from build123d import *

# Parameters (mm, degrees)
F0_W      = 368.3
F0_H      = 50.8
F1_DEPTH  = 38.1
F2_W      = 76.2
F2_H      = 50.8
F3_DEPTH  = 38.1
F4_W      = 3.175
F4_H      = 63.5
F5_DEPTH  = 12.7
F6_W      = 44.45
F6_H      = 50.8
F7_DEPTH  = 38.1
F8_R      = 2.54
F9_DEPTH  = 12.7
F10_W     = 76.2
F10_H     = 6.35
F10_W_2   = 38.1
F11_DEPTH = 76.2


with BuildPart() as f1:
    # F0 (on Right) → F1 (new body)
    with BuildSketch(Plane.YZ):
        with Locations((184.15, 25.4)):
            Rectangle(F0_W, F0_H)
    extrude(amount=F1_DEPTH)

    # F2 (on face) → F3 (join)
    with BuildSketch(Plane.YZ.offset(38.1)):
        with Locations((38.1, 25.4)):
            Rectangle(F2_W, F2_H)
        with Locations((330.2, 25.4)):
            Rectangle(F2_W, F2_H)
    extrude(amount=F3_DEPTH)

    # F4 (on face) → F5 (cut)
    with BuildSketch(Plane.XY.offset(50.8)):
        with Locations((13.5509, 38.1)):
            Rectangle(F4_W, F4_H)
        with Locations((13.5509, 330.2)):
            Rectangle(F4_W, F4_H)
        Polygon((10.905067, 69.85), (11.9634, 69.85), (15.1384, 69.85), (15.1384, 298.45), (11.9634, 298.45), (10.905067, 298.45), align=None)
    extrude(amount=-F5_DEPTH, mode=Mode.SUBTRACT)

    # F6 (on face) → F7 (cut)
    with BuildSketch(Plane.XY.offset(50.8)):
        with Locations((47.625, 38.1)):
            Rectangle(F6_W, F6_H)
        with Locations((47.625, 330.2)):
            Rectangle(F6_W, F6_H)
    extrude(amount=-F7_DEPTH, mode=Mode.SUBTRACT)

    # F8 (on face) → F9 (cut)
    with BuildSketch(Plane.YZ.offset(38.1)):
        with Locations((120.65, 25.4)):
            Circle(F8_R)
        with Locations((146.05, 25.4)):
            Circle(F8_R)
        with Locations((171.45, 25.4)):
            Circle(F8_R)
        with Locations((196.85, 25.4)):
            Circle(F8_R)
        with Locations((222.25, 25.4)):
            Circle(F8_R)
        with Locations((247.65, 25.4)):
            Circle(F8_R)
        with Locations((95.25, 25.4)):
            Circle(F8_R)
        with Locations((273.05, 25.4)):
            Circle(F8_R)
    extrude(amount=-F9_DEPTH, mode=Mode.SUBTRACT)

    # F10 (on face) → F11 (cut)
    with BuildSketch(Plane.XY.offset(50.8)):
        with Locations((38.1, 3.175)):
            Rectangle(F10_W, F10_H)
        with Locations((57.15, 73.025)):
            Rectangle(F10_W_2, F10_H)
        with Locations((38.1, 365.125)):
            Rectangle(F10_W, F10_H)
        with Locations((57.15, 295.275)):
            Rectangle(F10_W_2, F10_H)
    extrude(amount=-F11_DEPTH, mode=Mode.SUBTRACT)


solid = f1.part
CAD build for the part. Positions are in the model's coordinates, mm. A direction names the side the tool comes from. Coordinates: 2 decimals unless noted, no trailing zeros. Order: outer loops, then holes, each group sorted by start corner. A loop starts at its lowest first (then second) coordinate and runs counter-clockwise, first axis right, second up. Notation, with made-up numbers: (-7.5, 43.25) -> (-2.5, 43.25) arc R7 cw to (-2.5, 55.25) -> close; hole circle Ø11 at (56, 49.25). An arc over 180 degrees is marked (long way). Answer in a Markdown table with one row per item.
1) Band-saw the part on B-B (y = 29). List the corners of the cut face in (x, z).
Check values:
| item | result |
|---|---|
| outline | (0, 0) -> (76.2, 0) -> (76.2, 50.8) -> (69.85, 50.8) -> (69.85, 12.7) -> (25.4, 12.7) -> (25.4, 50.8) -> (15.14, 50.8) -> (15.14, 38.1) -> (11.96, 38.1) -> (11.96, 50.8) -> (0, 50.8) -> close |
2) Mould opens along Y. For faces 1 (the face through (11.963, 330, 45)), 2 (the face through (38, 361.95, 26)), 3 (the face through (10.905, 186, 45)) say: pulls with the +Y half, pulls with the -Y half, needs draft (parallel to the pull), parting line crosses it, or undercut.
Check values:
| item | result |
|---|---|
| face 1 | needs draft |
| face 2 | pulls with the +Y half |
| face 3 | undercut |
3) Drill centre lines: line 1 (Y direction, x = 40, z = 24.5); line 2 (Y direction, x = 25.5, z = 46.5); line 3 (Z direction, x = 35.75, y = 120.65). Where is each one in solid material? Low to high.
Check values:
| item | result |
|---|---|
| line 1 | 6.35 to 12.7, 63.5 to 69.85, 298.45 to 304.8, 355.6 to 361.95 |
| line 2 | 6.35 to 12.7, 63.5 to 304.8, 355.6 to 361.95 |
| line 3 | 0 to 22.86, 27.94 to 50.8 |
4) Which spindle directions (+Z, -Z, +X, -X, +Y, -Y) get a long thin tool onto all of the face, cutting with end or side? Do faces 4 (the face through (47, 355.6, 32)), 5 (the face through (6, 182, 50.8)), 6 (the face through (38.1, 183, 26)). Say none if no direction does.
Check values:
| item | result |
|---|---|
| face 4 | +Z |
| face 5 | +Z, +X, -X, +Y, -Y |
| face 6 | +Z, -Z, +X |
5) Band-saw the part on A-A (x = 48.5). List the corners of the cut face in (y, z), and give its area (3 significant figures).
Check values:
| item | result |
|---|---|
| outline | (6.35, 0) -> (69.85, 0) -> (69.85, 50.8) -> (63.5, 50.8) -> (63.5, 12.7) -> (12.7, 12.7) -> (12.7, 50.8) -> (6.35, 50.8) -> close; (298.45, 0) -> (361.95, 0) -> (361.95, 50.8) -> (355.6, 50.8) -> (355.6, 12.7) -> (304.8, 12.7) -> (304.8, 50.8) -> (298.45, 50.8) -> close |
| area | 2,580 mm2 |
6) Flat gauge pins, fed straight in: P1, Ø5.5, axis at y = 121.5, z = 26, coming from the +X side; P2, Ø1.5, axis at x = 35, y = 48, coming from the +Z side; P3, Ø3, axis at y = 171.45, z = 25.4, coming from the +X side. Where does each tip first touch, or does it go through?
Check values:
| item | result |
|---|---|
| P1 | x = 38.1 |
| P2 | z = 12.7 |
| P3 | x = 25.4 |
7) Band-saw the part on C-C (y = 295). List the corners of the cut face in (x, z).
Check values:
| item | result |
|---|---|
| outline | (0, 0) -> (38.1, 0) -> (38.1, 50.8) -> (15.14, 50.8) -> (15.14, 38.1) -> (10.91, 38.1) -> (10.91, 50.8) -> (0, 50.8) -> close |
